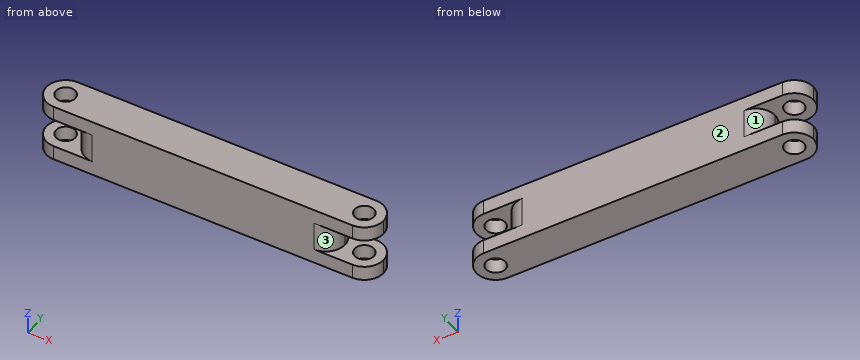
```python
from build123d import *

# Parameters (mm, degrees)
Y_KSEKLIK_EKSTR_ZYON1_DEPTH = 40
KES_EKSTR_ZYON1_REACH       = 191.275
IZIM2_R                     = 10
RADYUS1_R                   = 20


with BuildPart() as part:
    # Çizim1 → Yükseklik-Ekstrüzyon1 (new body)
    with BuildSketch(Plane(origin=(0, 0, 0), x_dir=(1, 0, 0), z_dir=(0, 1, 0))):
        Polygon((-135, -15), (-135, 15), (-175, 15), (-175, 30), (175, 30), (175, 15), (135, 15), (135, -15), (175, -15), (175, -30), (-175, -30), (-175, -15), align=None)
    extrude(amount=-Y_KSEKLIK_EKSTR_ZYON1_DEPTH)

    # Kes-Ekstrüzyon1: up to this face of the body (flat: up to its plane)
    kes_ekstr_zyon1_end = Plane(part.part.faces().sort_by_distance((0, -20, -30))[0])
    # Çizim2 → Kes-Ekstrüzyon1 (cut, up to the picked face)
    with BuildSketch(Plane.XY.offset(30), mode=Mode.PRIVATE) as kes_ekstr_zyon1_sk1:
        with Locations((-155, -20)):
            Circle(IZIM2_R)
    kes_ekstr_zyon1_tool1 = split(extrude(kes_ekstr_zyon1_sk1.sketch, amount=-KES_EKSTR_ZYON1_REACH, mode=Mode.PRIVATE), bisect_by=kes_ekstr_zyon1_end, keep=Keep.BOTH, mode=Mode.PRIVATE)
    # Çizim2 → Kes-Ekstrüzyon1 (cut, up to the picked face)
    with BuildSketch(Plane.XY.offset(30), mode=Mode.PRIVATE) as kes_ekstr_zyon1_sk2:
        with Locations(Location((155, -20, 0), (0, 0, 180))):
            Circle(IZIM2_R)
    kes_ekstr_zyon1_tool2 = split(extrude(kes_ekstr_zyon1_sk2.sketch, amount=-KES_EKSTR_ZYON1_REACH, mode=Mode.PRIVATE), bisect_by=kes_ekstr_zyon1_end, keep=Keep.BOTH, mode=Mode.PRIVATE)
    add(kes_ekstr_zyon1_tool1.solids().sort_by(Axis((-155, -20, 30), (0, 0, -1)))[0], mode=Mode.SUBTRACT)
    add(kes_ekstr_zyon1_tool2.solids().sort_by(Axis((155, -20, 30), (0, 0, -1)))[0], mode=Mode.SUBTRACT)

    # Radyus1
    radyus1_edges = [part.edges().sort_by_distance(p)[0] for p in [
        (135, -40, 0),
        (135, 0, 0),
        (-135, -40, 0),
        (-135, 0, 0),
        (-175, -40, -22.5),
        (-175, 0, -22.5),
        (-175, 0, 22.5),
        (-175, -40, 22.5),
        (175, 0, -22.5),
        (175, -40, -22.5),
        (175, -40, 22.5),
        (175, 0, 22.5),
    ]]
    fillet(radyus1_edges, radius=RADYUS1_R - 0.0001)  # a hair under: the kernel refuses the full size


solid = part.part
```
Part model, mm, in its own coordinate system. Face numbers are marked on the shaded views. A direction names the side the tool comes from. Round coordinates to 2 decimals unless told otherwise and drop trailing zeros. Write each loop counter-clockwise with the first axis right and the second up, starting at its lowest first coordinate (ties: lowest second). Pieces come first, ordered by that corner, then holes. Notation, with made-up numbers: (-40, -9) -> (0, -9) arc R26 cw to (0, 12) -> close; hole circle Ø3 at (-2.75, 30). An arc over 180 degrees is marked (long way). Return JSON: item names as keys, results as strings. Group by question number.
Q1. Pin check, flat tips, straight feed: pin 1 (16 mm diameter, centred on x = 155, y = -20, fed in from +Z); pin 2 (1 mm diameter, centred on y = -35, z = 23.5, fed in from +X); pin 3 (10 mm diameter, centred on x = 121.5, z = 9.5, fed in from +Y); pin 4 (2 mm diameter, centred on y = -35.5, z = -1, fed in from -X). Stop position of each tip, or through.
Q2. Probe L1, parallel to Y at x = 155, z = -24; L2, parallel to X at y = -21.5, z = -17.5; L3, parallel to X at y = -13, z = 26.5. List the from-to ranges inside material, lowest first. Write a range as [from, to].
Q3. Saw through at D-D on x = 120.5. Write the cut outline in (y, z).
Q4. Which spindle directions (+Z, -Z, +X, -X, +Y, -Y) get a long thin tool onto all of the face, cutting with end or side? Do the marked faces 1, 2 and 3. Say none if no direction does.
Q5. Saw through at C-C on y = -4.5. Write the cut outline in (x, z), plus the area to 3 significant figures.
Q6. Saw through at B-B on x = -151. Write the cut outline in (y, z), plus the area to 3 significant figures.
Answer:
{
 "1": {"pin 1": "through", "pin 2": "x = 168.78", "pin 3": "y = -0.06", "pin 4": "x = -128.78"},
 "2": {"L1": "[-40, -30], [-10, 0]", "L2": "[-174.94, -164.89], [-145.11, 145.11], [164.89, 174.94]", "L3": "[-173.74, -162.14], [-147.86, 147.86], [162.14, 173.74]"},
 "3": {"outline": "(-40, -30) -> (0, -30) -> (0, -15) -> (-0.77, -15) -> (-0.77, 15) -> (0, 15) -> (0, 30) -> (-40, 30) -> (-40, 15) -> (-39.23, 15) -> (-39.23, -15) -> (-40, -15) -> close"},
 "4": {"face 1": "-X, +Y", "face 2": "+Z, -Z, +X, -X, +Y", "face 3": "+X, -Y"},
 "5": {"outline": "(-167.64, -30) -> (167.64, -30) -> (167.64, -15) -> (127.64, -15) -> (127.64, 15) -> (167.64, 15) -> (167.64, 30) -> (-167.64, 30) -> (-167.64, 15) -> (-127.64, 15) -> (-127.64, -15) -> (-167.64, -15) -> close", "area": "17,700 mm2"},
 "6": {"outline": "(-40, -30) -> (-29.17, -30) -> (-29.17, -15) -> (-40, -15) -> close; (-40, 15) -> (-29.17, 15) -> (-29.17, 30) -> (-40, 30) -> close; (-10.83, -30) -> (0, -30) -> (0, -15) -> (-10.83, -15) -> close; (-10.83, 15) -> (0, 15) -> (0, 30) -> (-10.83, 30) -> close", "area": "650 mm2"}
}
